from build123d import *

# Parameters (mm, degrees)
F0_W     = 40
F0_H     = 40
F1_DEPTH = 40
F2_W     = 20
F2_H     = 20
F3_DEPTH = 20
F7_DEPTH = 24.4958974278


with BuildPart() as f1:
    # F0 (on Front) → F1 (new body)
    with BuildSketch(Plane.XZ):
        with Locations((20, 20)):
            Rectangle(F0_W, F0_H)
    extrude(amount=F1_DEPTH)

    # F2 (on face) → F3 (cut)
    with BuildSketch(Plane.XZ.offset(40)):
        with Locations((30, 30)):
            Rectangle(F2_W, F2_H)
    extrude(amount=-F3_DEPTH, mode=Mode.SUBTRACT)

    # F6 (on 3pt) → F7 (cut, through all)
    with BuildSketch(Plane(origin=(16.6666666667, -16.6666666667, 33.3333333333), x_dir=(0.9128709292, 0.1825741858, -0.3651483717), z_dir=(-0.4082482905, 0.4082482905, -0.8164965809))):
        Polygon((3.6514837167, 26.83281573), (25.5603860169, 8.94427191), (25.5603860169, 31.304951685), align=None)
    extrude(amount=-F7_DEPTH, mode=Mode.SUBTRACT)

    # F9 (on 3pt) → F10 (join, up to the next surface of F1)
    with BuildSketch(Plane(origin=(26.6666666667, -26.6666666667, 26.6666666667), x_dir=(-0.4082482905, -0.8164965809, -0.4082482905), z_dir=(-0.5773502692, 0.5773502692, -0.5773502692))):
        Polygon((16.3299316186, 0), (-8.1649658093, 14.1421356237), (-8.1649658093, -14.1421356237), align=None)
    extrude(until=Until.NEXT)


solid = f1.part
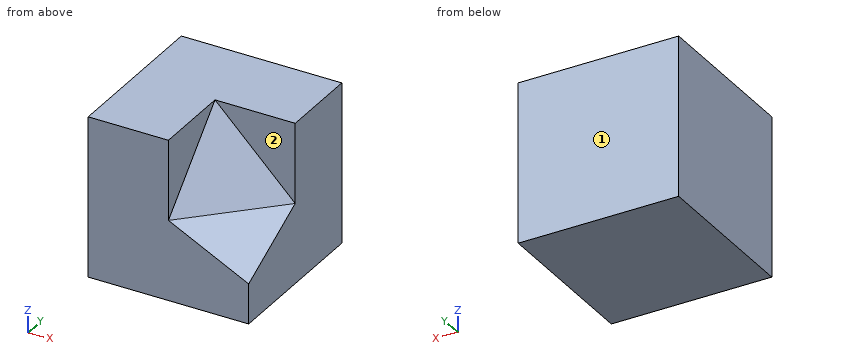
Verification items for the finished model (mm, model axes). Face numbers are marked on the shaded views. A direction names the side the tool comes from. Coordinates: 2 decimals unless noted, no trailing zeros. Order: outer loops, then holes, each group sorted by start corner. A loop starts at its lowest first (then second) coordinate and runs counter-clockwise, first axis right, second up. Notation, with made-up numbers: (59.25, 7.25) -> (89.25, 7.25) arc R26 cw to (89.25, 43.25) -> close; hole circle Ø5 at (-9, 2.25). An arc over 180 degrees is marked (long way). Put each result on its own line as item: value. Start each with the question number.
1. Go/stop test with flat-tipped pins: pin 1 Ø10 at (x, y) = (14, -29.5) entering from -Z; pin 2 Ø8 at (y, z) = (-35, 35.5) entering from +X. Record where each tip stops, or that it passes through.
2. Cross-section at B-B, the plane z = 25. Record the boundary of the cut face in (x, y).
3. Cross-section at C-C, the plane z = 19. Record the boundary of the cut face in (x, y), then the cut area to 3 significant figures.
4. Cross-section at A-A, the plane y = -21. Record the boundary of the cut face in (x, z).
5. Material ranges on L1, parallel to Z at x = 27.5, y = -20.5; L2, parallel to Y at x = 26.5, z = 18; L3, parallel to Y at x = 36, z = 17, recorded low to high. Write a range as [from, to].
6. Access from +Z, -Z, +X, -X, +Y, -Y to the whole of each face (thin tool, end or side, straight path). Record for the marked faces 1 and 2.
Computed:
1. pin 1: z = 0
1. pin 2: x = 20
2. outline: (0, -40) -> (20, -40) -> (20, -35) -> (35, -20) -> (40, -20) -> (40, 0) -> (0, 0) -> close
3. outline: (0, -40) -> (22, -40) -> (40, -22) -> (40, 0) -> (0, 0) -> close
3. area: 1,440 mm2
4. outline: (0, 0) -> (40, 0) -> (40, 19.5) -> (39, 20) -> (20, 39) -> (20, 40) -> (0, 40) -> close
5. L1: [0, 32]
5. L2: [-37.5, 0]
5. L3: [-30, 0]
6. face 1: +Z, -Z, +X, -X, +Y
6. face 2: +Z, +X, -Y
